from build123d import *

# Parameters (mm, degrees)
SKETCH_1_W          = 67.6
SKETCH_1_H          = 50
EXTRUDE_1_DEPTH     = 7
SKETCH_2_R          = 2
CUT_EXTRUDE_1_DEPTH = 10
SKETCH_3_W          = 47.6
SKETCH_3_H          = 40
CUT_EXTRUDE_2_DEPTH = 7
FILLET_1_R          = 2


with BuildPart() as part:
    # 草图1 → 凸台-拉伸1 (new body)
    with BuildSketch(Plane.XY):
        with Locations((33.8, 25)):
            Rectangle(SKETCH_1_W, SKETCH_1_H)
    extrude(amount=EXTRUDE_1_DEPTH)

    # 草图2 → 切除-拉伸1 (cut)
    with BuildSketch(Plane.ZY):
        with Locations((3.5, 40)):
            Circle(SKETCH_2_R)
        with Locations((3.5, 30)):
            Circle(SKETCH_2_R)
        with Locations((3.5, 20)):
            Circle(SKETCH_2_R)
        with Locations((3.5, 10)):
            Circle(SKETCH_2_R)
    cut_extrude_1 = extrude(amount=-CUT_EXTRUDE_1_DEPTH, mode=Mode.SUBTRACT)

    # 镜向1: 切除-拉伸1 across plane
    add(cut_extrude_1.mirror(Plane(origin=(33.8, 0, 0), x_dir=(0, 0, 1), z_dir=(1, 0, 0))), mode=Mode.SUBTRACT)

    # 草图3 → 切除-拉伸2 (cut)
    with BuildSketch(Plane.XY.offset(7)):
        with Locations((33.8, 25)):
            Rectangle(SKETCH_3_W, SKETCH_3_H)
    extrude(amount=-CUT_EXTRUDE_2_DEPTH, mode=Mode.SUBTRACT)

    # 圆角1
    fillet_1_edges = [part.edges().sort_by_distance(p)[0] for p in [
        (10, 5, 3.5),
        (10, 45, 3.5),
        (57.6, 45, 3.5),
        (57.6, 5, 3.5),
    ]]
    fillet(fillet_1_edges, radius=FILLET_1_R)


solid = part.part
The model under review builds one solid part; all positions refer to its coordinate system, in mm. A direction names the side the tool comes from. Coordinates: 2 decimals unless noted, no trailing zeros. Loops run counter-clockwise (first coordinate to the right, second up) from the corner with the lowest first, then second, coordinate; pieces in that order, holes last. Notation, with made-up numbers: M 88,31 L 112,31 A20 cw 112,55 Z; hole C 77,81.5 d3. An arc over 180 degrees is marked long. Put each result on its own line as item: value. Start each with the question number.
Q1. Wall thickness on line 1 (Y direction, x = 61.5, z = 3.5); line 2 (X direction, y = 32.5, z = 5.5); line 3 (Y direction, x = 32, z = 5.5): over which ranges is each line inside the solid? List them lowest first.
Q2. Add section B-B (y = 17). Write out the cut boundary in (x, z).
Q3. Add section A-A (x = 23). Write out the cut boundary in (y, z).
Q4. For faces 1 (the cylindrical face through (4.93, 21.983, 3.24)), 2 (the flat face through (57.6, 25, 4)), list the 3-axis set-ups (+Z, -Z, +X, -X, +Y, -Y) from which the entire face can be reached by the end or side of a thin tool; tool diameter is ignored.
Q5. Add section C-C (y = 30). Write out the cut boundary in (x, z), and give its area (3 significant figures).
Q6. The part is to be moulded in two halves that separate along Z. For faces 3 (the cylindrical face through (10.6, 5.57, 3.45)), 4 (the cylindrical face through (4.93, 28.048, 3.066)), 5 (the cylindrical face through (62.67, 28.048, 3.066)), 6 (the flat face through (33, 3, 7)), say which applies: +Z half, -Z half, draft (parallel to the pull), parting line (faces both ways), or undercut.
Q7. Add section D-D (z = 3.5). Count the separate pieces of the cut face and the enclosed holes in it, and give its area (3 significant figures).
Answers:
1. line 1: y = 0 to 8, 12 to 18, 22 to 28, 32 to 38, 42 to 50
1. line 2: x = 0 to 10, 57.6 to 67.6
1. line 3: y = 0 to 5, 45 to 50
2. outline: M 0,0 L 10,0 L 10,7 L 0,7 Z; M 57.6,0 L 67.6,0 L 67.6,7 L 57.6,7 Z
3. outline: M 0,0 L 5,0 L 5,7 L 0,7 Z; M 45,0 L 50,0 L 50,7 L 45,7 Z
4. face 1: +X, -X
4. face 2: +Z, -Z
5. outline: M 0,0 L 10,0 L 10,1.5 L 0,1.5 Z; M 0,5.5 L 10,5.5 L 10,7 L 0,7 Z; M 57.6,0 L 67.6,0 L 67.6,1.5 L 57.6,1.5 Z; M 57.6,5.5 L 67.6,5.5 L 67.6,7 L 57.6,7 Z
5. area: 60.0 mm^2
6. face 3: draft
6. face 4: undercut
6. face 5: undercut
6. face 6: +Z half
7. separate pieces: 8
7. enclosed holes: 0
7. area: 1,160 mm^2
